The listing builds one solid part. Answer for the finished solid, in the listing's coordinates (mm). Give positions to 0.01 mm unless a question says otherwise; leave off trailing zeros. Order: outer loops, then holes, each group sorted by start corner. A loop starts at its lowest first (then second) coordinate and runs counter-clockwise, first axis right, second up. Notation, with made-up numbers: (-36, 40.5) - (-17, 40.5) arc R15 ccw to (-17, 63.5) - close; hole circle Ø6 at (40, 32). An arc over 180 degrees is marked (long way). Write each question's results on one line, items separated by ' | '. Start each with the question number.
1. Flat-ended cylindrical pins translate along their axes: pin 1 (1 mm diameter, centred on x = 19, z = 5, fed in from +Y); pin 2 (3 mm diameter, centred on x = 8.5, y = 5, fed in from +Z). Find the tip coordinate at first contact, or state that the pin passes through.
2. Section C-C (z = 8.25) is taken. Give the vertices of the cut face in (x, y).
3. Section A-A (y = 5) is taken. Give the vertices of the cut face in (x, z).
4. Section B-B (x = 35.25) is taken. Give the vertices of the cut face in (y, z).
5. Find the intervals of material crossed by L1, parallel to X at y = 23, z = 9.05; L2, parallel to X at y = 69, z = 1.85; L3, parallel to Z at x = 12.5, y = 67, in increasing order.
6. Section D-D (y = 58) is taken. Give the vertices of the cut face in (x, z).
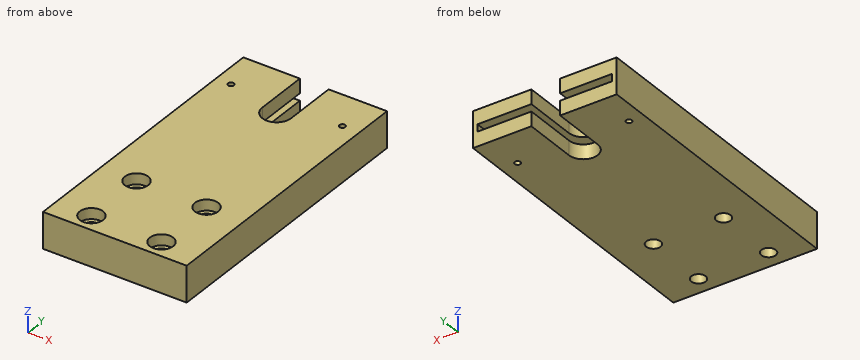
Autodesk Fusion 360 part; units mm, degrees
sketch "Sketch1" plane through (0, 0, 0) normal (0, 0, 1) x (1, 0, 0)
  line L0 (0, 0) -> (40, 0)
  line L1 (40, 0) -> (40, 80)
  line L2 (40, 80) -> (0, 80)
  line L3 (0, 80) -> (0, 0)
  line L4 (10, 5) -> (29.5, 5)
  line L5 (29.5, 5) -> (29.5, 23)
  line L6 (29.5, 23) -> (10, 23)
  line L7 (10, 23) -> (10, 5)
  line L8 (19.75, 23) -> (19.75, 65)
  circle A0 centre (19.75, 65) radius 4
  circle A1 centre (10, 23) radius 2
  circle A2 centre (10, 5) radius 2
  circle A3 centre (29.5, 23) radius 2
  circle A4 centre (29.5, 5) radius 2
  line L9 (15.75, 65) -> (15.75, 80)
  line L10 (23.75, 65) -> (23.75, 80)
  line L11 (19.75, 61) -> (35.25, 61)
  line L12 (19.75, 61) -> (4.25, 61)
  line L13 (35.25, 61) -> (35.25, 69)
  circle A5 centre (35.25, 69) radius 0.8
  line L14 (4.25, 61) -> (4.25, 69)
  circle A6 centre (4.25, 69) radius 0.8
  dimension "d1" = 40
  dimension "d2" = 80
  dimension "d3" = 19.5
  dimension "d4" = 18
  dimension "d6" = 42
  dimension "d7" = 8
  dimension "d8" = 4
  dimension "d9" = 4
  dimension "d10" = 4
  dimension "d11" = 4
  dimension "d22" = 15.5
  dimension "d23" = 15.5
  dimension "d24" = 8
  dimension "d25" = 1.6
  dimension "d26" = 8
  dimension "d27" = 1.6
extrude "Extrude1" add sketch "Sketch1" along normal blind 10 contours L4 L5 L6 L7 A1 A2 A3 A4 | L0 L1 L2 L3 A0 L9 L10
sketch "Sketch3" plane through (0, 80, 0) normal (0, 1, 0) x (-1, 0, 0)
  line L0 (-40, 0) -> (-23.75, 0)
  line L1 (-23.75, 0) -> (-23.75, 10)
  line L2 (-23.75, 10) -> (-40, 10)
  line L3 (-40, 10) -> (-40, 0)
  line L4 (-40, 0) -> (-40, 4)
  line L5 (-40, 4) -> (-40, 6)
  line L6 (-40, 6) -> (-40, 10)
  line L7 (-20, 4) -> (-20, 6)
  line L8 (-20, 5) -> (-1.25, 5)
  line L9 (-20, 5) -> (-38.75, 5)
  line L10 (-38.75, 5) -> (-38.75, 6)
  line L11 (-1.25, 5) -> (-1.25, 4)
  line L12 (-38.75, 6) -> (-1.25, 6)
  line L13 (-1.25, 6) -> (-1.25, 4)
  line L14 (-1.25, 4) -> (-38.75, 4)
  line L15 (-38.75, 4) -> (-38.75, 6)
  dimension "d14" = 4
  dimension "d15" = 2
  dimension "d16" = 18.75
  dimension "d17" = 18.75
  dimension "d18" = 1
  dimension "d19" = 1
extrude "Extrude2" cut sketch "Sketch3" against normal blind 31 contours L1 L9 L14 L15 | L1 L7 L9 L14 | L1 L9 L10 L12 L15 | L1 L7 L9 L12 | L7 L8 L11 L13 L14 | L7 L8 L12 L13
sketch "Sketch4" plane through (0, 49, 0) normal (0, 1, 0) x (-1, 0, 0)
  line L0 (-1.25, 6) -> (-38.75, 6)
  line L1 (-38.75, 6) -> (-38.75, 4)
  line L2 (-38.75, 4) -> (-1.25, 4)
  line L3 (-1.25, 4) -> (-1.25, 6)
  line L4 (-22.5, 6) -> (-17.5, 6)
  line L5 (-17.5, 6) -> (-17.5, 4)
  line L6 (-17.5, 4) -> (-22.5, 4)
  line L7 (-22.5, 4) -> (-22.5, 6)
  dimension "d30" = 5
  dimension "d31" = 2
extrude "Extrude3" cut sketch "Sketch4" against normal blind 6 contours L0 L2 L4 L5 L6 L7
sketch "Sketch5" plane through (0, 0, 10) normal (0, 0, 1) x (-1, 0, 0)
  circle A0 centre (-10, -23) radius 2
  circle A1 centre (-29.5, -5) radius 2
  circle A2 centre (-35.25, -69) radius 0.8
  circle A3 centre (-4.25, -69) radius 0.8
  circle A4 centre (-29.5, -23) radius 2
  circle A5 centre (-10, -5) radius 2
  line L0 (-15.75, -65) -> (-15.75, -80)
  line L1 (-15.75, -80) -> (0, -80)
  line L2 (0, -80) -> (0, 0)
  line L3 (0, 0) -> (-40, 0)
  line L4 (-40, 0) -> (-40, -80)
  line L5 (-40, -80) -> (-23.75, -80)
  line L6 (-23.75, -80) -> (-23.75, -65)
  arc A6 (-15.75, -65) -> (-23.75, -65) centre (-19.75, -65) ccw
  circle A7 centre (-10, -5) radius 3.25
  circle A8 centre (-10, -23) radius 3.25
  circle A9 centre (-29.5, -5) radius 3.25
  circle A10 centre (-29.5, -23) radius 3.25
  dimension "d34" = 6.5
  dimension "d35" = 6.5
  dimension "d36" = 6.5
  dimension "d37" = 6.5
extrude "Extrude4" cut sketch "Sketch5" against normal blind 3 contours A7 | A8 | A9 | A10
Reported:
1) pin 1: y = 43 | pin 2: z = 7
2) outline: (0, 0) - (40, 0) - (40, 80) - (23.75, 80) - (23.75, 65) arc R4 cw to (15.75, 65) - (15.75, 80) - (0, 80) - close; hole circle Ø1.6 at (4.25, 69); hole circle Ø6.5 at (10, 5); hole circle Ø6.5 at (10, 23); hole circle Ø6.5 at (29.5, 5); hole circle Ø6.5 at (29.5, 23); hole circle Ø1.6 at (35.25, 69)
3) outline: (0, 0) - (8, 0) - (8, 7) - (6.75, 7) - (6.75, 10) - (0, 10) - close; (12, 0) - (27.5, 0) - (27.5, 7) - (26.25, 7) - (26.25, 10) - (13.25, 10) - (13.25, 7) - (12, 7) - close; (31.5, 0) - (40, 0) - (40, 10) - (32.75, 10) - (32.75, 7) - (31.5, 7) - close
4) outline: (0, 0) - (68.2, 0) - (68.2, 4) - (49, 4) - (49, 6) - (68.2, 6) - (68.2, 10) - (0, 10) - close; (69.8, 0) - (80, 0) - (80, 4) - (69.8, 4) - close; (69.8, 6) - (80, 6) - (80, 10) - (69.8, 10) - close
5) L1: 0 to 6.75, 13.25 to 26.25, 32.75 to 40 | L2: 0 to 3.45, 5.05 to 15.75, 23.75 to 34.45, 36.05 to 40 | L3: 0 to 4, 6 to 10
6) outline: (0, 0) - (40, 0) - (40, 10) - (0, 10) - close; hole (1.25, 4) - (38.75, 4) - (38.75, 6) - (1.25, 6) - close
